Work out the finished part from the listing and answer in its coordinate system (mm). Face numbers are marked on the shaded views. A direction names the side the tool comes from. Round coordinates to 2 decimals unless told otherwise and drop trailing zeros. Order: outer loops, then holes, each group sorted by start corner. A loop starts at its lowest first (then second) coordinate and runs counter-clockwise, first axis right, second up. Notation, with made-up numbers: M 4,15 L 16,15 A20 ccw 16,27 Z; hole C 58.5,50.5 d11. An arc over 180 degrees is marked long. Return JSON: item names as keys, results as strings.
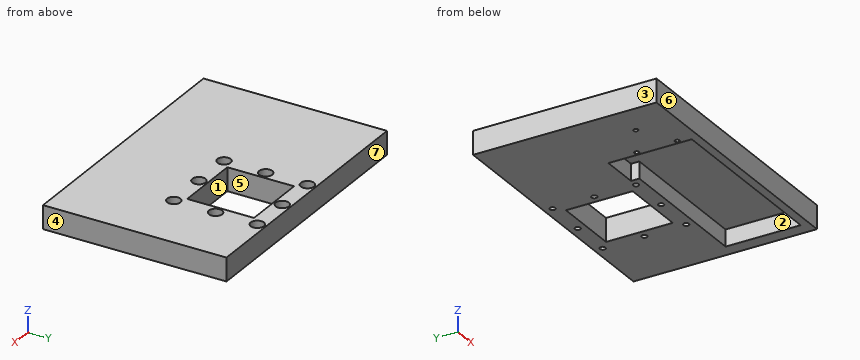
Autodesk Inventor part; units mm, degrees
ref_plane "YZ Plane" through (0, 0, 0) normal (1, 0, 0) x (0, 1, 0)
ref_plane "XZ Plane" through (0, 0, 0) normal (0, 1, 0) x (-1, 0, 0)
ref_plane "XY Plane" through (0, 0, 0) normal (0, 0, 1) x (1, 0, 0)
ref_plane "Work Plane1" through (0, 0, 0) normal (0, 0, 1) x (1, 0, 0)
sketch "Sketch1" plane through (0, 0, 0) normal (0, 0, 1) x (1, 0, 0)
  circle A0 centre (0, 25) radius 1.95 construction
  circle A1 centre (-25, 0) radius 1.95 construction
  circle A2 centre (-25, -25) radius 1.95 construction
  circle A3 centre (25, 25) radius 1.95 construction
  circle A4 centre (25, -25) radius 1.95 construction
  circle A5 centre (-25, 25) radius 1.95 construction
  circle A6 centre (25, 0) radius 1.95 construction
  circle A7 centre (0, -25) radius 1.95 construction
  line L0 (-28, 30) -> (-30, 28) construction
  line L1 (-30, 28) -> (-30, -28) construction
  line L2 (-30, -28) -> (-28, -30) construction
  line L3 (-28, -30) -> (28, -30) construction
  line L4 (28, -30) -> (30, -28) construction
  line L5 (30, -28) -> (30, 28) construction
  line L6 (30, 28) -> (28, 30) construction
  line L7 (28, 30) -> (-28, 30) construction
  circle A8 centre (35, -56) radius 1 construction
  circle A9 centre (5, -48.5) radius 1 construction
  circle A10 centre (5, -64.5) radius 1.0474 construction
  circle A11 centre (-5, -64.5) radius 1 construction
  circle A12 centre (-5, -56) radius 1 construction
  circle A13 centre (-5, -48.5) radius 1 construction
  circle A14 centre (5, -56) radius 1 construction
  circle A15 centre (35, -48) radius 1 construction
  circle A16 centre (35, -64) radius 1 construction
  line L8 (38, -40) -> (38, -72) construction
  line L9 (38, -40) -> (-10, -40) construction
  line L10 (-10, -72) -> (-10, -40) construction
  line L11 (38, -72) -> (-10, -72) construction
  line L12 (38, -71) -> (38, -41) construction
  line L13 (38, -71) -> (48, -71) construction
  line L14 (48, -41) -> (48, -71) construction
  line L15 (38, -41) -> (48, -41) construction
  line L16 (56, -75) -> (-52.5, -75)
  line L17 (-52.5, -75) -> (-52.5, -30)
  line L18 (-52.5, -30) -> (56, -30)
  line L19 (56, -30) -> (56, -75)
  line L20 (-40, -41.1445) -> (-40, -68) construction
  line L21 (-41, -39.0927) -> (-41, -47.7587) construction
  line L22 (-41, -39.0927) -> (-46.5, -39.0927) construction
  line L23 (-46.5, -47.7587) -> (-46.5, -39.0927) construction
  line L24 (-41, -47.7587) -> (-46.5, -47.7587) construction
  line L25 (-41, -60.5) -> (-41, -64) construction
  line L26 (-41, -60.5) -> (-46.5, -60.5) construction
  line L27 (-46.5, -64) -> (-46.5, -60.5) construction
  line L28 (-41, -64) -> (-46.5, -64) construction
  line L29 (64, 30) -> (-96, 30)
  line L30 (-96, 30) -> (-96, -80)
  line L31 (-96, -80) -> (64, -80)
  line L32 (64, -80) -> (64, 30)
  line L33 (20, -20) -> (-20, -20)
  line L34 (-20, -20) -> (-20, 20)
  line L35 (-20, 20) -> (20, 20)
  line L36 (20, 20) -> (20, -20)
  line L37 (20, -20) -> (-20, 20) construction
  line L38 (-20, -20) -> (20, 20) construction
  line L39 (-52.5, -30) -> (-30, -30)
  line L40 (-30, -30) -> (-30, -25)
  line L41 (-30, -25) -> (-52.5, -25)
  line L42 (-52.5, -25) -> (-52.5, -30)
  point P0 (0, 0)
  dimension "d1" = 3
  dimension "d2" = 8
  dimension "d4" = 6
  dimension "d5" = 160
  dimension "d6" = 110
  dimension "d7" = 8
  dimension "d19" = 40
  dimension "d20" = 40
  dimension "d28" = 5
  dimension "d29" = 0
extrude "Extrusion1" add sketch "Sketch1" along normal blind 10
sketch "Sketch2" plane through (0, 0, 10) normal (0, 0, 1) x (1, 0, 0)
  line L0 (-30, -30) -> (56, -30)
  line L1 (56, -30) -> (56, -75)
  line L2 (56, -75) -> (-52.5, -75)
  line L3 (64, 30) -> (-96, 30)
  line L4 (-96, 30) -> (-96, -80)
  line L5 (-96, -80) -> (64, -80)
  line L6 (64, -80) -> (64, 30)
  line L7 (20, -20) -> (20, 20)
  line L8 (-20, -20) -> (20, -20)
  line L9 (20, -20) -> (20, 20)
  line L10 (20, 20) -> (-20, 20)
  line L11 (-20, 20) -> (-20, -20)
  line L12 (-20, -20) -> (20, 20) construction
  line L13 (20, -20) -> (-20, 20) construction
  line L14 (-52.5, -25) -> (-30, -25)
  line L15 (-30, -25) -> (-30, -30)
  line L16 (-52.5, -75) -> (-52.5, -25)
  point P0 (0, 0)
extrude "Extrusion2" add sketch "Sketch2" along normal blind 4 contours L0 L1 L2 L16 L14 L15 | L6 L5 L4 L3
sketch "Sketch3" plane through (0, 0, 14) normal (0, 0, 1) x (1, 0, 0)
  circle A0 centre (0, 25) radius 1.95 construction
  circle A1 centre (-25, 0) radius 1.95 construction
  circle A2 centre (-25, -25) radius 1.95 construction
  circle A3 centre (25, 25) radius 1.95 construction
  circle A4 centre (25, -25) radius 1.95 construction
  circle A5 centre (-25, 25) radius 1.95 construction
  circle A6 centre (25, 0) radius 1.95 construction
  circle A7 centre (0, -25) radius 1.95 construction
  line L0 (-28, 30) -> (-30, 28) construction
  line L1 (-30, 28) -> (-30, -28) construction
  line L2 (-30, -28) -> (-28, -30) construction
  line L3 (-28, -30) -> (28, -30) construction
  line L4 (28, -30) -> (30, -28) construction
  line L5 (30, -28) -> (30, 28) construction
  line L6 (30, 28) -> (28, 30) construction
  line L7 (28, 30) -> (-28, 30) construction
  point P0 (0, 0)
hole "Hole1" at (25, 25, 14) at (0, 25, 14) at (-25, 25, 14) at (-25, 0, 14) at (-25, -25, 14) at (0, -25, 14) at (25, -25, 14) at (25, 0, 14) direction (0, 0, -1) diameter 3.3 end through all counterbore diameter 8 counterbore depth 5
sketch "Sketch4" plane through (0, 0, 0) normal (0, 0, -1) x (-1, 0, 0)
  line L0 (52.5, -75) -> (-56, -75) construction
  line L1 (-56, -75) -> (-56, -30) construction
  line L2 (-56, -30) -> (30, -30) construction
  line L3 (20, 20) -> (20, -20) construction
  line L4 (20, -20) -> (-20, -20) construction
  line L5 (-20, -20) -> (-20, 20) construction
  line L6 (-20, 20) -> (20, 20) construction
  line L7 (-64, 30) -> (96, 30) construction
  line L8 (-64, -80) -> (-64, 30) construction
  line L9 (96, -80) -> (-64, -80) construction
  line L10 (96, 30) -> (96, -80) construction
  line L11 (54.8114, -67.6244) -> (54.8114, -43.3756) construction
  line L12 (54.8114, -43.3756) -> (75.8114, -55.5) construction
  line L13 (75.8114, -55.5) -> (54.8114, -67.6244) construction
  line L14 (96, 30) -> (96, -80) construction
  line L15 (30, -30) -> (30, -25)
  line L16 (30, -25) -> (52.5, -25)
  line L17 (52.5, -25) -> (52.5, -75)
  line L18 (20, -49.5) -> (16.4, -49.5)
  line L19 (20, -61.5) -> (16.4, -61.5)
  circle A0 centre (5, -55.5) radius 1.8
  point P0 (0, 0)
  point P1 (61.8114, -55.5)
  dimension "d30" = 21
  dimension "d31" = 0
hole "Hole2" at (-54.8114, -43.3756, 0) at (-75.8114, -55.5, 0) at (-54.8114, -67.6244, 0) direction (0, 0, 1) diameter 2.8 depth 12 tip angle 118
properties part number "cellSTORM_Base_v0"
Item 1: Each of these flat-tipped pins is pushed along its axis until it touches: pin 1 (6.5 mm diameter, centred on x = 0, y = 25, fed in from +Z); pin 2 (2 mm diameter, centred on x = 7.5, y = -31.5, fed in from -Z); pin 3 (2 mm diameter, centred on x = 0, y = -25, fed in from -Z). Where does it stop, or does it pass through?
Output:
{"pin 1": "stops at z = 9", "pin 2": "stops at z = 10", "pin 3": "passes through"}
Item 2: Find section A-A (x = 25). State how many separate pieces and enclosed holes the cut face has, plus the area to 3 significant figures.
Output:
{"separate pieces": "4", "enclosed holes": "0", "area": "881 mm^2"}
Item 3: Find section B-B (y = 17.5). Determine the outline of the cut face in (x, z).
Output:
{"outline": "M -96,0 L -20,0 L -20,14 L -96,14 Z; M 20,0 L 64,0 L 64,14 L 20,14 Z"}
Item 4: Find section D-D (x = 0). Determine the outline of the cut face in (y, z), plus the area to 3 significant figures.
Output:
{"outline": "M -80,0 L -75,0 L -75,10 L -30,10 L -30,0 L -26.65,0 L -26.65,9 L -29,9 L -29,14 L -80,14 Z; M -23.35,0 L -20,0 L -20,14 L -21,14 L -21,9 L -23.35,9 Z; M 20,0 L 23.35,0 L 23.35,9 L 21,9 L 21,14 L 20,14 Z; M 26.65,0 L 30,0 L 30,14 L 29,14 L 29,9 L 26.65,9 Z", "area": "391 mm^2"}
Item 5: Which of the six approach directions +Z, -Z, +X, -X, +Y, -Y give full straight-line access (tool end or side, diameter ignored) to the marked faces 1, 2 and 3?
Output:
{"face 1": "+Z, -Z", "face 2": "-Z", "face 3": "+Z, -Z, -X, +Y, -Y"}
Item 6: The mould has two halves that part along Y. Classify the marked faces 4, 5, 6 and 7: pulls with the +Y half, pulls with the -Y half, needs draft (parallel to the pull), parting line crosses it, or undercut.
Output:
{"face 4": "needs draft", "face 5": "undercut", "face 6": "pulls with the -Y half", "face 7": "pulls with the +Y half"}
Item 7: Consider line 1 along X through (y, z) = (25, 5.25); line 2 along Y through (x, z) = (25, 6.5); line 3 along Y through (x, z) = (25, 10.35). Determine where each line is inside the solid, lowest interval first. Write a range as [from, to].
Output:
{"line 1": "x = [-96, -26.65], [-23.35, -1.65], [1.65, 23.35], [26.65, 64]", "line 2": "y = [-80, -75], [-30, -26.65], [-23.35, -1.65], [1.65, 23.35], [26.65, 30]", "line 3": "y = [-80, -29], [-21, -4], [4, 21], [29, 30]"}
Item 8: Find section C-C (y = 0). Determine the outline of the cut face in (x, z), plus the area to 3 significant figures.
Output:
{"outline": "M -96,0 L -26.65,0 L -26.65,9 L -29,9 L -29,14 L -96,14 Z; M -23.35,0 L -20,0 L -20,14 L -21,14 L -21,9 L -23.35,9 Z; M 20,0 L 23.35,0 L 23.35,9 L 21,9 L 21,14 L 20,14 Z; M 26.65,0 L 64,0 L 64,14 L 29,14 L 29,9 L 26.65,9 Z", "area": "1,540 mm^2"}
